Geometry: final body of the model. Coordinates: model frame, mm. A direction names the side the tool comes from. Coordinates: 2 decimals unless noted, no trailing zeros. Write each loop counter-clockwise with the first axis right and the second up, starting at its lowest first coordinate (ties: lowest second). Pieces come first, ordered by that corner, then holes. Notation, with made-up numbers: (56, 33) -> (97, 33) arc R17 cw to (97, 47) -> close; hole circle Ø9 at (40, 20). An arc over 180 degrees is marked (long way). One line per item, written item: value.
```python
from build123d import *

# Parameters (mm, degrees)
EXTRUDE_THIN1_DEPTH     = 101.6
FILLET1_R               = 25.4
FILLET2_R               = 25.4
CUT_EXTRUDE1_DEPTH      = 15.494
CUT_EXTRUDE1_DEPTH_BACK = 67.818
CUT_EXTRUDE2_DEPTH      = 20.32
CUT_EXTRUDE2_DEPTH_BACK = 16.51
SKETCH3_R               = 1.5875
CUT_EXTRUDE3_DEPTH      = 14.732
CUT_EXTRUDE3_DEPTH_BACK = 22.86
SKETCH4_R               = 1.5875


with BuildPart() as part:
    # Sketch1 → Extrude-Thin1 (new, symmetric)
    with BuildSketch(Plane.XY):
        with BuildLine():
            Line((0, 0), (-19.05, 0))
            ThreePointArc((-19.05, 0), (-37.010512242, 7.439487758), (-44.45, 25.4))
            Line((-44.45, 25.4), (-44.45, 342.9))
            Line((-44.45, 342.9), (-36.83, 342.9))
            Line((-36.83, 342.9), (-36.83, 25.4))
            ThreePointArc((-36.83, 25.4), (-31.622358569, 12.827641431), (-19.05, 7.62))
            Line((-19.05, 7.62), (0, 7.62))
            Line((0, 7.62), (0, 0))
        make_face()
    extrude(amount=EXTRUDE_THIN1_DEPTH, both=True)

    # Fillet1
    fillet1_edges = [part.edges().sort_by_distance(p)[0] for p in [
        (-40.64, 342.9, 101.6),
    ]]
    fillet(fillet1_edges, radius=FILLET1_R)

    # Fillet2
    fillet2_edges = [part.edges().sort_by_distance(p)[0] for p in [
        (-40.64, 342.9, -101.6),
    ]]
    fillet(fillet2_edges, radius=FILLET2_R)

    # Sketch2 → Cut-Extrude1 (cut, two sides: drawn at the far end of the back side and taken through both)
    with BuildSketch(Plane(origin=(0, 0, 0), x_dir=(0, 0, -1), z_dir=(1, 0, 0)).offset(-CUT_EXTRUDE1_DEPTH_BACK)):
        with BuildLine():
            Line((-101.6, 0), (-76.2, 0))
            ThreePointArc((-76.2, 0), (-83.132124101, 22.895250599), (-101.6, 38.1))
            Line((-101.6, 38.1), (-101.6, 0))
        make_face()
        with BuildLine():
            Line((101.6, 0), (101.6, 38.1))
            ThreePointArc((101.6, 38.1), (83.132124101, 22.895250599), (76.2, 0))
            Line((76.2, 0), (101.6, 0))
        make_face()
    extrude(amount=CUT_EXTRUDE1_DEPTH + CUT_EXTRUDE1_DEPTH_BACK, mode=Mode.SUBTRACT)

    # Sketch3 → Cut-Extrude2 (cut, two sides: drawn at the far end of the back side and taken through both)
    with BuildSketch(Plane(origin=(-36.83, 0, 0), x_dir=(0, 0, -1), z_dir=(1, 0, 0)).offset(-CUT_EXTRUDE2_DEPTH_BACK)):
        with Locations(Location((-76.2, 279.4, 0), (0, 0, 180))):
            Circle(SKETCH3_R)
        with Locations(Location((76.2, 279.4, 0), (0, 0, 180))):
            Circle(SKETCH3_R)
    extrude(amount=CUT_EXTRUDE2_DEPTH + CUT_EXTRUDE2_DEPTH_BACK, mode=Mode.SUBTRACT)

    # Sketch4 → Cut-Extrude3 (cut, two sides: drawn at the far end of the back side and taken through both)
    with BuildSketch(Plane(origin=(0, 7.62, 0), x_dir=(1, 0, 0), z_dir=(0, 1, 0)).offset(-CUT_EXTRUDE3_DEPTH_BACK)):
        with Locations(Location((-19.05, -50.8, 0), (0, 0, 270))):
            Circle(SKETCH4_R)
        with Locations(Location((-19.05, 50.8, 0), (0, 0, 270))):
            Circle(SKETCH4_R)
    extrude(amount=CUT_EXTRUDE3_DEPTH + CUT_EXTRUDE3_DEPTH_BACK, mode=Mode.SUBTRACT)


solid = part.part
```
(1) Reachability of faces 1 (the flat face through (-9, 0, 1)), 2 (the flat face through (-36.83, 186, 1)) from +Z, -Z, +X, -X, +Y, -Y: full face, straight path, thin tool, end or side. Return the list, or none.
Responses:
face 1: +Z, -Z, +X, -X, -Y
face 2: +Z, -Z, +X, +Y
(2) Line query: line 1 (Z direction, x = -40.25, y = 279.4); line 2 (Z direction, x = -19.05, y = 3.5); line 3 (X direction, y = 69, z = -67.5). Output: solid intervals per line, ascending. Write a range as [from, to].
Responses:
line 1: z = [-101.6, -77.79], [-74.61, 74.61], [77.79, 101.6]
line 2: z = [-76.35, -52.39], [-49.21, 49.21], [52.39, 76.35]
line 3: x = [-44.45, -36.83]
(3) Section B-B (y = 223). Return the cut outline in (x, z).
Responses:
outline: (-44.45, -101.6) -> (-36.83, -101.6) -> (-36.83, 101.6) -> (-44.45, 101.6) -> close
(4) First-contact query: pin 1 (5.5 mm diameter, centred on x = -8.5, z = -28.5, fed in from +Y); pin 2 (12 mm diameter, centred on x = -22, z = 52.5, fed in from +Y); pin 3 (5 mm diameter, centred on x = -19.05, z = -50.8, fed in from +Y). Flat tips, straight axial feed; report the tip coordinate or a pass-through.
Responses:
pin 1: stops at y = 7.62
pin 2: stops at y = 10.04
pin 3: stops at y = 7.8
(5) Section A-A (z = 61). Return the cut outline in (x, y).
Responses:
outline: (-44.45, 25.4) arc R25.4 ccw to (-19.05, 0) -> (0, 0) -> (0, 7.62) -> (-19.05, 7.62) arc R17.78 cw to (-36.83, 25.4) -> (-36.83, 342.9) -> (-44.45, 342.9) -> close
